Check sheet for the modelled part. Datum: model origin and axes. Units: mm. Face numbers are marked on the shaded views. Coordinates: 2 decimals unless noted, no trailing zeros. Loops run counter-clockwise (first coordinate to the right, second up) from the corner with the lowest first, then second, coordinate; pieces in that order, holes last. Notation, with made-up numbers: (72.25, 22.25) -> (103.25, 22.25) arc R12 ccw to (103.25, 37.25) -> close; hole circle Ø6 at (-5.75, -31.75). An arc over 180 degrees is marked (long way). Use one line per item in the form item = value.
from build123d import *

# Parameters (mm, degrees)
SKETCH1_W           = 16
SKETCH1_H           = 16
SKETCH1_W_2         = 14
SKETCH1_H_2         = 14
BOSS_EXTRUDE1_DEPTH = 169
SKETCH2_R           = 4.25
SKETCH2_R_2         = 1.5
CUT_EXTRUDE1_DEPTH  = 170.944108459


# Read off the part's stored shape, not the designer's step: CSK for M3 Flat Head Machine Screw1
with BuildPart() as part:
    # Sketch1 → Boss-Extrude1 (new body)
    with BuildSketch(Plane.XY):
        Rectangle(SKETCH1_W, SKETCH1_H)
        Rectangle(SKETCH1_W_2, SKETCH1_H_2, mode=Mode.SUBTRACT)
    extrude(amount=-BOSS_EXTRUDE1_DEPTH)

    # Sketch2 → Cut-Extrude1 (cut, through all)
    with BuildSketch(Plane(origin=(0, 8, 0), x_dir=(1, 0, 0), z_dir=(0, 1, 0))):
        with Locations(Location((0, 159.5, 0), (0, 0, 270))):
            Circle(SKETCH2_R)
        with Locations(Location((0, 9.5, 0), (0, 0, 270))):
            Circle(SKETCH2_R)
        with Locations(Location((0, 20.5, 0), (0, 0, 270))):
            Circle(SKETCH2_R_2)
        with Locations(Location((0, 148.5, 0), (0, 0, 270))):
            Circle(SKETCH2_R_2)
    extrude(amount=-CUT_EXTRUDE1_DEPTH, mode=Mode.SUBTRACT)

    # CSK for M3 Flat Head Machine Screw1 outl → CSK for M3 Flat Head Machine Screw1 (revolve, cut)
    with BuildSketch(Plane.XY.offset(-148.5)):
        Polygon((1.5, -8), (3.15, -8), (2.15, -7), (1.5, -7), align=None)
        Polygon((3.15, 8), (1.5, 8), (1.5, 7), (2.15, 7), align=None)
    revolve(axis=Axis((0, 0, -148.5), (0, 1, 0)), mode=Mode.SUBTRACT)

    # CSK for M3 Flat Head Machine Screw1 2 ou → CSK for M3 Flat Head Machine Screw1 2 (revolve, cut)
    with BuildSketch(Plane.XY.offset(-20.5)):
        Polygon((1.5, -8), (3.15, -8), (2.15, -7), (1.5, -7), align=None)
        Polygon((3.15, 8), (1.5, 8), (1.5, 7), (2.15, 7), align=None)
    revolve(axis=Axis((0, 0, -20.5), (0, 1, 0)), mode=Mode.SUBTRACT)


solid = part.part
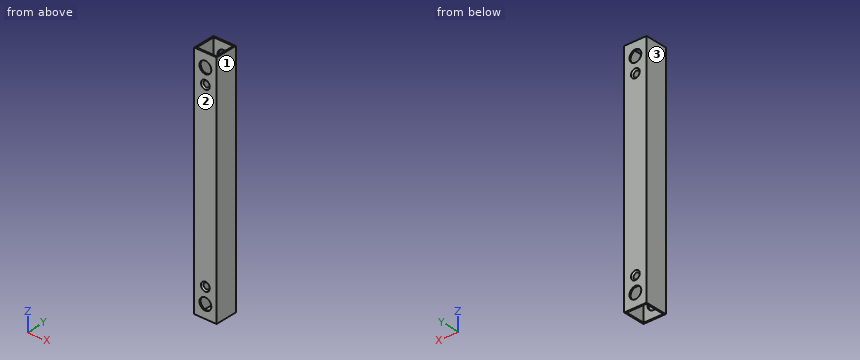
(1) Section check A-A, the plane y = 1. Record the boundary of the cut face in (x, z), plus the area to 3 significant figures.
Established:
outline = (-8, -169) -> (-7, -169) -> (-7, 0) -> (-8, 0) -> close; (7, -169) -> (8, -169) -> (8, 0) -> (7, 0) -> close
area = 338 mm²
(2) Section check C-C, the plane z = -105.5. Record the boundary of the cut face in (x, y).
Established:
outline = (-8, -8) -> (8, -8) -> (8, 8) -> (-8, 8) -> close; hole (-7, -7) -> (7, -7) -> (7, 7) -> (-7, 7) -> close
(3) Mould release check, pull along X, two halves, no side actions. Record for the marked faces 1, 2 and 3: +X half, -X half, draft (parallel to the pull), parting line (faces both ways), or undercut.
Established:
face_1 = +X half
face_2 = draft
face_3 = -X half
(4) Scan lines: line 1 along Y through (x, z) = (6, -79.5); line 2 along X through (y, z) = (7.85, -9.5). Record each from-to range of solid material in increasing order.
Established:
line_1 = -8 to -7, 7 to 8
line_2 = -8 to -4.25, 4.25 to 8
(5) Section check D-D, the plane x = 0. Give the number of separate pieces and of enclosed holes in the cut face, plus the area to 3 significant figures.
Established:
separate_pieces = 10
enclosed_holes = 0
area = 283 mm²
(6) Section check B-B, the plane z = -148.5. Record the boundary of the cut face in (x, y).
Established:
outline = (-8, -8) -> (-3.15, -8) -> (-2.15, -7) -> (-7, -7) -> (-7, 7) -> (-2.15, 7) -> (-3.15, 8) -> (-8, 8) -> close; (2.15, -7) -> (3.15, -8) -> (8, -8) -> (8, 8) -> (3.15, 8) -> (2.15, 7) -> (7, 7) -> (7, -7) -> close
